Geometry check sheet. Reference: drawing and pictorial views, mm from the part's lowest x, y, z. Round coordinates to 2 decimals unless told otherwise and drop trailing zeros. Loops run counter-clockwise (first coordinate to the right, second up) from the corner with the lowest first, then second, coordinate; pieces in that order, holes last. Notation, with made-up numbers: (27, 29.5) - (71, 29.5) arc R23 ccw to (71, 38.5) - close; hole circle Ø5 at (61, 15.25). An arc over 180 degrees is marked (long way). Answer as CSV lines item,"result". Start each with the question number.
1) Draft check along Y on the marked faces 1 and 2. Enter one of: released by +Y, released by -Y, zero draft, split by the parting line, or undercut.
2) Cross-section at C-C on z = 81.2. Record the boundary of the cut face in (x, y).
3) Depth check by flat-ended pin: P1, Ø6.5, axis at x = 87.7, z = 81.2, coming from the -Y side. Enter the tip coordinate at first touch or a pass-through.
4) Thickness scan on line 1 along X through (y, z) = (2.75, 12.7); line 2 along X through (y, z) = (4.75, 59.65); line 3 along Z through (x, y) = (87.7, 1.5). Record the ranges inside material, lowest first.
5) Cross-section at A-A on x = 87.7. Record the boundary of the cut face in (y, z).
6) Cross-section at B-B on y = 4.75. State how many separate pieces and enclosed holes the cut face has, and give its area (3 significant figures).
7) Cross-section at D-D on x = 37.5. Record the boundary of the cut face in (y, z).
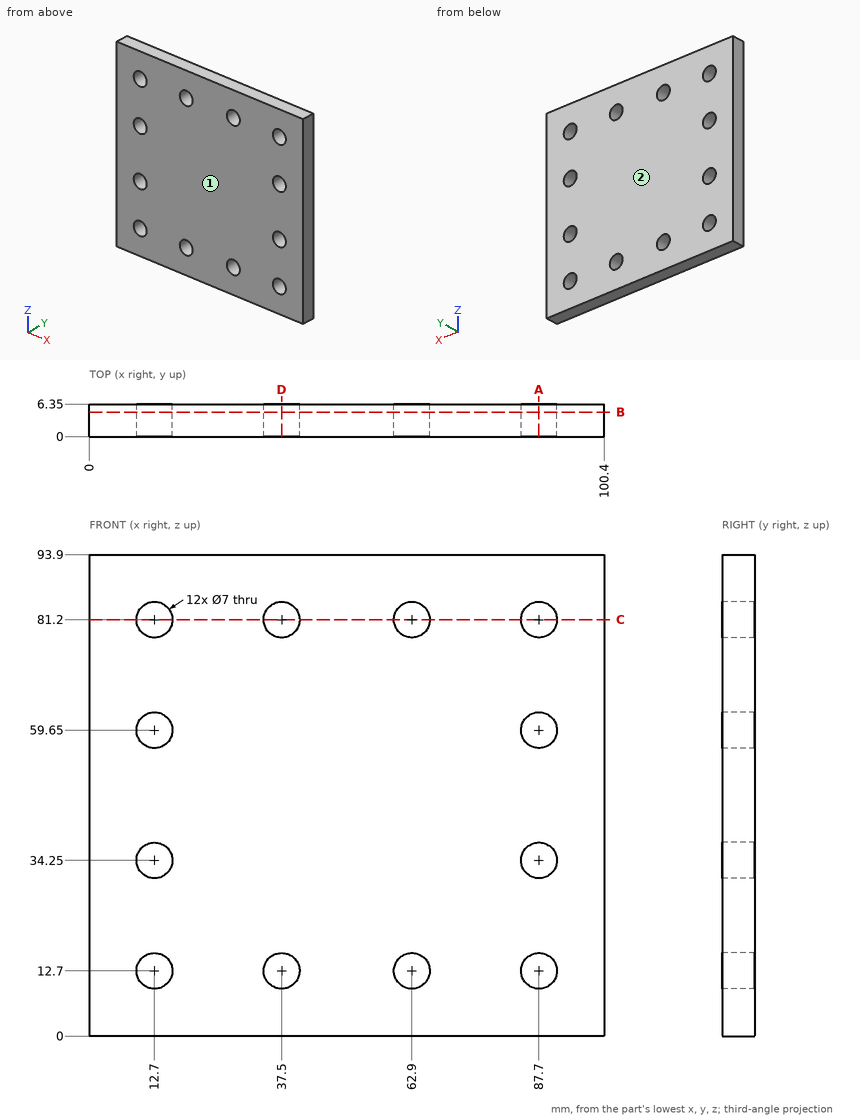
Answer block:
1,face 1,"released by -Y"
1,face 2,"released by +Y"
2,outline,"(0, 0) - (9.2, 0) - (9.2, 6.35) - (0, 6.35) - close; (16.2, 0) - (34, 0) - (34, 6.35) - (16.2, 6.35) - close; (41, 0) - (59.4, 0) - (59.4, 6.35) - (41, 6.35) - close; (66.4, 0) - (84.2, 0) - (84.2, 6.35) - (66.4, 6.35) - close; (91.2, 0) - (100.4, 0) - (100.4, 6.35) - (91.2, 6.35) - close"
3,P1,"passes through"
4,line 1,"x = 0 to 9.2, 16.2 to 34, 41 to 59.4, 66.4 to 84.2, 91.2 to 100.4"
4,line 2,"x = 0 to 9.2, 16.2 to 84.2, 91.2 to 100.4"
4,line 3,"z = 0 to 9.2, 16.2 to 30.75, 37.75 to 56.15, 63.15 to 77.7, 84.7 to 93.9"
5,outline,"(0, 0) - (6.35, 0) - (6.35, 9.2) - (0, 9.2) - close; (0, 16.2) - (6.35, 16.2) - (6.35, 30.75) - (0, 30.75) - close; (0, 37.75) - (6.35, 37.75) - (6.35, 56.15) - (0, 56.15) - close; (0, 63.15) - (6.35, 63.15) - (6.35, 77.7) - (0, 77.7) - close; (0, 84.7) - (6.35, 84.7) - (6.35, 93.9) - (0, 93.9) - close"
6,separate pieces,"1"
6,enclosed holes,"12"
6,area,"8,970 mm^2"
7,outline,"(0, 0) - (6.35, 0) - (6.35, 9.2) - (0, 9.2) - close; (0, 16.2) - (6.35, 16.2) - (6.35, 77.7) - (0, 77.7) - close; (0, 84.7) - (6.35, 84.7) - (6.35, 93.9) - (0, 93.9) - close"
